```python
from build123d import *

# Parameters (mm, degrees)
F0_W      = 133.35
F0_H      = 76.2
F1_DEPTH  = 42.672
F2_W      = 21.59
F2_H      = 4.572
F3_DEPTH  = 76.201
F5_DEPTH  = 42.673
F4_W      = 63.754
F4_H      = 76.2
F6_DEPTH  = 6.35
F3_FACE_W = 76.2
F3_FACE_H = 28.702
F7_DEPTH  = 9.398
F9_DEPTH  = 63.754
F10_R     = 14.224
F11_DEPTH = 36.323


with BuildPart() as f1:
    # F0 (on Top) → F1 (new body)
    with BuildSketch(Plane.XY):
        with Locations((-21.765223, 12.652185)):
            Rectangle(F0_W, F0_H)
    extrude(amount=F1_DEPTH)

    # F2 (on face) → F3 (cut, through all)
    with BuildSketch(Plane.XZ.offset(25.447815)):
        with Locations((-77.645223, 2.286)):
            Rectangle(F2_W, F2_H)
        Polygon((44.909777, 0), (44.909777, 33.274), (-24.686223, 33.274), (-24.686223, 4.572), (-46.276223, 4.572), (-46.276223, 0), align=None)
    extrude(amount=-F3_DEPTH, mode=Mode.SUBTRACT)

    # F4 (on face) → F5 (cut, through all)
    with BuildSketch(Plane.XY.offset(42.672)):
        Polygon((44.909777, 50.752185), (-1.064223, 50.752185), (44.909777, 17.351185), align=None)
        Polygon((44.909777, 7.953185), (-1.064223, -25.447815), (44.909777, -25.447815), align=None)
    extrude(amount=-F5_DEPTH, mode=Mode.SUBTRACT)

    # F4 (on face) → F6 (cut)
    with BuildSketch(Plane.XY.offset(42.672)):
        with Locations((-56.563223, 12.652185)):
            Rectangle(F4_W, F4_H)
    extrude(amount=-F6_DEPTH, mode=Mode.SUBTRACT)

    # F3_face (on face) → F7 (join)
    with BuildSketch(Plane(origin=(-24.686223, 12.652185, 18.923), x_dir=(0, 1, 0), z_dir=(1, 0, 0))):
        Rectangle(F3_FACE_W, F3_FACE_H)
    extrude(amount=F7_DEPTH)

    # F8 (on face) → F9 (cut)
    with BuildSketch(Plane(origin=(-88.440223, 0, 0), x_dir=(0, -1, 0), z_dir=(-1, 0, 0))):
        Polygon((-50.752185, 26.924), (-41.354185, 36.322), (-50.752185, 36.322), align=None)
        Polygon((25.447815, 36.322), (16.049815, 36.322), (25.447815, 26.924), align=None)
    extrude(amount=-F9_DEPTH, mode=Mode.SUBTRACT)

    # F10 (on face) → F11 (cut, through all)
    with BuildSketch(Plane.XY.offset(36.322)):
        with Locations((-56.690223, 12.652185)):
            Circle(F10_R)
    extrude(amount=-F11_DEPTH, mode=Mode.SUBTRACT)


solid = f1.part
```
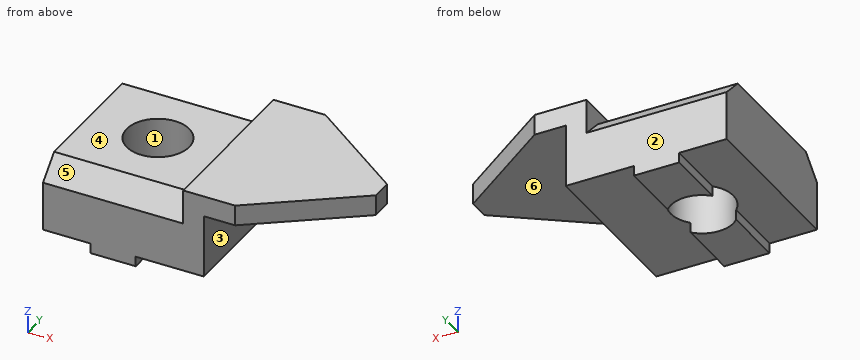
Design review of the part built by this model. Coordinates are the model's own, in mm. Face numbers are marked on the shaded views. A direction names the side the tool comes from. Coordinates: 2 decimals unless noted, no trailing zeros. Write each loop counter-clockwise with the first axis right and the second up, starting at its lowest first coordinate (ties: lowest second). Pieces come first, ordered by that corner, then holes.
1) Add section C-C (z = 29.5). Write out the cut boundary in (x, y), plus the area to 3 significant figures.
2) Add section D-D (y = 39). Write out the cut boundary in (x, z).
3) Add section A-A (y = 24). Write out the cut boundary in (x, z).
4) Mouldability with a two-part tool opening along X and no side actions: class the marked faces 1, 2 and 3 as +X half, -X half, draft (parallel to the pull), parting line (faces both ways), or undercut.
5) Insertion check: pin 1 (6.5 mm diameter, centred on x = -81.5, y = 3.5, fed in from -Z); pin 2 (5 mm diameter, centred on y = -6.5, z = 1.5, fed in from -X); pin 3 (23 mm diameter, centred on y = 2, z = 24.5, fed in from +X); pin 4 (1 mm diameter, centred on y = -13.5, z = 25, fed in from +X). Each pin has a flat end and moves straight along its axis. Give the tip position at first contact, or say it passes through.
6) Machinability: for the marked faces 4, 5 and 6, which of the approach directions +Z, -Z, +X, -X, +Y, -Y give a long, thin tool a straight path to every point of the face, cutting with its end or side? Answer none if there is none.
7) To check wall thickness, follow L1, parallel to Z at x = 4.5, y = 11; L2, parallel to Z at x = -21.5, y = 20.5; L3, parallel to X at y = 47.5, z = 4. State the ranges of each line that lie inside material, in increasing order.
8) Add section B-B (x = -52). Write out the cut boundary in (y, z).
Check result:
1. outline: (-88.44, -22.87) - (-24.69, -22.87) - (-24.69, -25.45) - (-15.29, -25.45) - (-15.29, 50.75) - (-24.69, 50.75) - (-24.69, 48.18) - (-88.44, 48.18) - close; hole circle Ø28.45 at (-56.69, 12.65)
1. area: 4,610 mm2
2. outline: (-88.44, 4.57) - (-66.85, 4.57) - (-66.85, 0) - (-46.28, 0) - (-46.28, 4.57) - (-15.29, 4.57) - (-15.29, 33.27) - (15.11, 33.27) - (15.11, 42.67) - (-24.69, 42.67) - (-24.69, 36.32) - (-88.44, 36.32) - close
3. outline: (-88.44, 4.57) - (-66.85, 4.57) - (-66.85, 0) - (-65.27, 0) - (-65.27, 36.32) - (-88.44, 36.32) - close; (-48.11, 0) - (-46.28, 0) - (-46.28, 4.57) - (-15.29, 4.57) - (-15.29, 33.27) - (35.76, 33.27) - (35.76, 42.67) - (-24.69, 42.67) - (-24.69, 36.32) - (-48.11, 36.32) - close
4. face 1: undercut
4. face 2: draft
4. face 3: +X half
5. pin 1: stops at z = 4.57
5. pin 2: stops at x = -66.85
5. pin 3: stops at x = 44.91
5. pin 4: stops at x = -15.29
6. face 4: +Z, -X, +Y, -Y
6. face 5: +Z, -X, -Y
6. face 6: -Z, +X, +Y, -Y
7. L1: z = 33.27 to 42.67
7. L2: z = 4.57 to 42.67
7. L3: x = -66.85 to -46.28
8. outline: (-25.45, 0) - (-0.78, 0) - (-0.78, 36.32) - (-16.05, 36.32) - (-25.45, 26.92) - close; (26.08, 0) - (50.75, 0) - (50.75, 26.92) - (41.35, 36.32) - (26.08, 36.32) - close
